CAD build for the part. Positions are in the model's coordinates, mm. Face numbers are marked on the shaded views. A direction names the side the tool comes from. Give positions to 0.01 mm unless a question says otherwise; leave off trailing zeros. Write each loop counter-clockwise with the first axis right and the second up, starting at its lowest first coordinate (ties: lowest second). Pieces come first, ordered by that corner, then holes. Notation, with made-up numbers: (21, 15) -> (58, 15) arc R19 cw to (58, 37) -> close; hole circle Ø9 at (68, 62). An arc over 180 degrees is marked (long way). Answer in a Markdown table with one row per item. Add a question column.
Autodesk Fusion 360 part; units mm, degrees
sketch "Sketch1" plane through (0, 0, 0) normal (0, 0, 1) x (1, 0, 0)
  line L0 (10, 13.5) -> (-10, 13.5)
  line L1 (-10, 13.5) -> (-10, -13.5)
  line L2 (-10, -13.5) -> (10, -13.5)
  line L3 (10, -13.5) -> (10, 13.5)
  line L4 (10, 13.5) -> (-10, -13.5) construction
  line L5 (-10, 13.5) -> (10, -13.5) construction
  circle A0 centre (0, 3.5) radius 2.5
  line L6 (-10, -13.5) -> (10, -13.5)
  line L7 (10, -13.5) -> (10, -7.5)
  line L8 (10, -7.5) -> (-10, -7.5)
  line L9 (-10, -7.5) -> (-10, -13.5)
  dimension "d1" = 20
  dimension "d2" = 27
  dimension "d3" = 5
  dimension "d4" = 10
  dimension "d5" = 6
extrude "Extrude1" add sketch "Sketch1" along normal blind 6 contours L0 L1 L3 L8
extrude "Extrude2" add sketch "Sketch1" along normal blind 20 contours L1 L2 L3 L6 L7 L8 L9
sketch "Sketch2" plane through (0, -13.5, 0) normal (0, -1, 0) x (1, 0, 0)
  line L0 (-10, 0) -> (10, 0)
  line L1 (10, 0) -> (10, 20)
  line L2 (10, 20) -> (-10, 20)
  line L3 (-10, 20) -> (-10, 0)
  circle A0 centre (0, 15) radius 2.5
  dimension "d10" = 5
  dimension "d11" = 15
extrude "Extrude3" cut sketch "Sketch2" against normal blind 90 contours A0
chamfer "Chamfer1" distance 5 distance2 4 1 edges at (0, -7.5, 6) measured on face at (-0.0623, -4.6643, 6)
fillet "Fillet1" radius 5 4 edges at (10, 13.5, 3) (-10, 13.5, 3) (-10, -10.5, 20) (10, -10.5, 20)
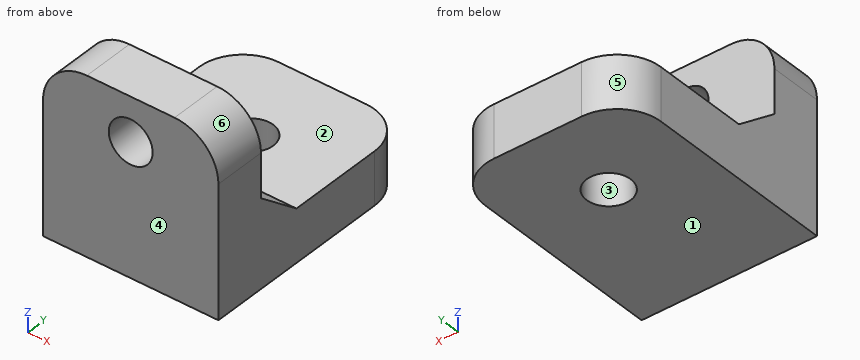
Item 1: Slice it at B-B, the plane x = 0. List the corners of the cut face in (y, z), then the cut area to 3 significant figures.
Item 2: Drop flat-ended pins along their axis: pin 1 Ø5 at (x, y) = (0.5, 3) entering from +Z; pin 2 Ø10 at (x, z) = (5, 16.5) entering from +Y; pin 3 Ø4 at (x, z) = (0, 15) entering from +Y. Give the stop position or say it passes through.
Item 3: Which spindle directions (+Z, -Z, +X, -X, +Y, -Y) get a long thin tool onto all of the face, cutting with end or side? Do the marked faces 1 and 2. Say none if no direction does.
Item 4: Slice it at A-A, the plane y = 3.5. List the corners of the cut face in (x, z).
Item 5: Slice it at C-C, the plane y = -11.5. List the corners of the cut face in (x, z), then the cut area to 3 significant figures.
Item 6: Mould opens along Y. For the marked faces 3, 4, 5 and 6 say: released by +Y, released by -Y, zero draft, split by the parting line, or undercut.
Item 7: Slice it at D-D, the plane x = -4. List the corners of the cut face in (y, z).
Item 8: Probe L1, parallel to Z at x = 0, y = -11.4; L2, parallel to Y at x = 9.25, z = 16.5; L3, parallel to X at y = 4.25, z = 5. List the from-to ranges inside material, lowest first. Write a range as from..to.
Answer key:
| question | item | result |
|---|---|---|
| 1 | outline | (-13.5, 0) -> (1, 0) -> (1, 6) -> (-2.5, 6) -> (-7.5, 10) -> (-7.5, 12.5) -> (-13.5, 12.5) -> close; (-13.5, 17.5) -> (-7.5, 17.5) -> (-7.5, 20) -> (-13.5, 20) -> close; (6, 0) -> (13.5, 0) -> (13.5, 6) -> (6, 6) -> close |
| 1 | area | 196 mm² |
| 2 | pin 1 | stops at z = 6 |
| 2 | pin 2 | stops at y = -7.5 |
| 2 | pin 3 | passes through |
| 3 | face 1 | -Z, +X, -X, +Y, -Y |
| 3 | face 2 | +Z, +X, -X, +Y |
| 4 | outline | (-10, 0) -> (-2.5, 0) -> (-2.5, 6) -> (-10, 6) -> close; (2.5, 0) -> (10, 0) -> (10, 6) -> (2.5, 6) -> close |
| 5 | outline | (-10, 0) -> (10, 0) -> (10, 15) arc R5 ccw to (5, 20) -> (-5, 20) arc R5 ccw to (-10, 15) -> close; hole circle Ø5 at (0, 15) |
| 5 | area | 370 mm² |
| 6 | face 3 | undercut |
| 6 | face 4 | released by -Y |
| 6 | face 5 | released by +Y |
| 6 | face 6 | zero draft |
| 7 | outline | (-13.5, 0) -> (13.5, 0) -> (13.5, 6) -> (-2.5, 6) -> (-7.5, 10) -> (-7.5, 20) -> (-13.5, 20) -> close |
| 8 | L1 | z = 0..12.5, 17.5..20 |
| 8 | L2 | y = -13.5..-7.5 |
| 8 | L3 | x = -10..-2.38, 2.38..10 |
